Autodesk Inventor part; units mm, degrees
ref_plane "YZ Plane" through (0, 0, 0) normal (1, 0, 0) x (0, 1, 0)
ref_plane "XZ Plane" through (0, 0, 0) normal (0, 1, 0) x (-1, 0, 0)
ref_plane "XY Plane" through (0, 0, 0) normal (0, 0, 1) x (1, 0, 0)
sketch "Sketch1" plane through (0, 0, 0) normal (0, 0, 1) x (1, 0, 0)
  line L0 (-20, -12) -> (20, -12)
  line L1 (20, -12) -> (20, 12)
  line L2 (20, 12) -> (-20, 12)
  line L3 (-20, 12) -> (-20, -12)
  line L4 (-20, -12) -> (20, 12) construction
  line L5 (20, -12) -> (-20, 12) construction
  point P0 (0, 0)
  dimension "d0" = 40
  dimension "d1" = 24
extrude "Extrusion1" add sketch "Sketch1" along normal blind 45
sketch "Sketch2" plane through (0, 0, 45) normal (0, 0, 1) x (1, 0, 0)
  line L0 (-20, -6) -> (-19.2, -6)
  line L1 (-19.2, -6) -> (-19.2, 6)
  line L2 (-19.2, 6) -> (-20, 6)
  line L3 (-20, 6) -> (-20, -6)
  line L4 (20, -12) -> (20, 12)
  line L5 (20, -6) -> (19.2, -6)
  line L6 (19.2, -6) -> (19.2, 6)
  line L7 (19.2, 6) -> (20, 6)
  line L8 (20, 6) -> (20, -6)
  point P0 (0, 0)
  point P1 (-20, 12)
  point P2 (-19.2, 0)
  point P3 (19.2, 0)
  dimension "d4" = 12
  dimension "d5" = 0.8
  dimension "d6" = 0.8
extrude "Extrusion2" add sketch "Sketch2" along normal blind 2.5
sketch "Sketch3" plane through (20, -12, 0) normal (1, 0, 0) x (0, 0, -1)
  line L0 (-47.5, 6) -> (-47.5, 18)
  line L1 (-47.5, 18) -> (-46.7, 18)
  line L2 (-46.7, 18) -> (-46.7, 6)
  line L3 (-46.7, 6) -> (-47.5, 6)
  line L4 (-47.5, 6) -> (-47.5, 18)
  point P0 (0, 12)
  dimension "d9" = 0.8
extrude "Extrusion3" add sketch "Sketch3" along normal blind 14
sketch "Sketch4" plane through (-20, -12, 0) normal (-1, 0, 0) x (0, 0, 1)
  line L0 (47.5, 18) -> (47.5, 6)
  line L1 (45, 18) -> (47.5, 18)
  line L2 (47.5, 6) -> (46.7, 6)
  line L3 (46.7, 6) -> (46.7, 18)
  line L4 (46.7, 18) -> (47.5, 18)
  line L5 (47.5, 18) -> (47.5, 6)
  point P0 (0, 12)
  dimension "d12" = 0.8
extrude "Extrusion4" add sketch "Sketch4" along normal blind 14
sketch "Sketch5" plane through (0, 0, 47.5) normal (0, 0, 1) x (1, 0, 0)
  line L0 (-28, 0) -> (28, 0) construction
  point P0 (0, 0)
  point P1 (0, 0)
  dimension "d15" = 56
hole "Hole1" at (-28, 0, 47.5) at (28, 0, 47.5) direction (0, 0, -1) diameter 5.5 end through all
fillet "Fillet1" radius 1 2 edges at (19.2, 0, 47.5) (-19.2, 0, 47.5)
properties part number "Snmubber"
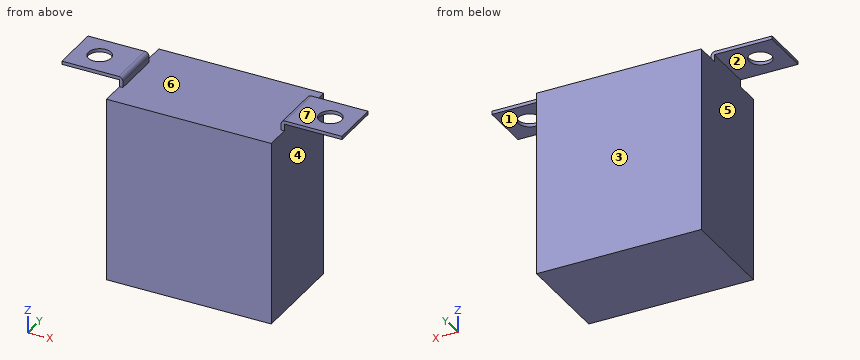
The listing builds one solid part. Answer for the finished solid, in the listing's coordinates (mm). Face numbers are marked on the shaded views. A direction names the side the tool comes from. Give positions to 0.01 mm unless a question says otherwise; leave off trailing zeros. Order: outer loops, then holes, each group sorted by start corner. A loop starts at its lowest first (then second) coordinate and runs counter-clockwise, first axis right, second up. Notation, with made-up numbers: (13, -10) - (40, -10) arc R12 cw to (40, 11) - close; hole circle Ø4 at (38, 54.25). An arc over 180 degrees is marked (long way). Answer in a Markdown table with one row per item. Add a question column.
Q1. The part is cut by section A-A (x = -28). Determine the outline of the cut face in (y, z), then the cut area to 3 significant figures.
Q2. The part is cut by section D-D (z = 41). Determine the outline of the cut face in (x, y).
Q3. Which of the six approach directions +Z, -Z, +X, -X, +Y, -Y give full straight-line access (tool end or side, diameter ignored) to the marked faces 1, 2 and 3?
Q4. For a pull along X with two mould halves and no side action, classify the marked faces 4, 5, 6 and 7 as released by +X, released by -X, zero draft, split by the parting line, or undercut.
Q5. The part is cut by section B-B (y = 0). Determine the outline of the cut face in (x, z), then the cut area to 3 significant figures.
Q6. Find the intervals of material crossed by line 1 along X through (y, z) = (0, 47.25); line 2 along Y through (x, z) = (28, 47.1); line 3 along X through (y, z) = (0, 47.1), in increasing order. Write a range as [from, to].
Q7. The part is cut by section C-C (y = -4.75). Determine the outline of the cut face in (x, z).
Q8. Given P1, Ø12, axis at y = -5.5, z = 23, coming from the +X side; P2, Ø0.8, axis at x = 23.5, z = 46, coming from the +Y side (1 decimal); P3, Ø7, axis at x = 28, y = 0, coming from the -Z side; P4, Ø12, axis at y = -1.5, z = 21, coming from the -X side, each flat-ended and moving along its own axis, determine where each tip first touches the part or whether it passes through.
Determined:
| question | item | result |
|---|---|---|
| 1 | outline | (-6, 46.7) - (-2.75, 46.7) - (-2.75, 47.5) - (-6, 47.5) - close; (2.75, 46.7) - (6, 46.7) - (6, 47.5) - (2.75, 47.5) - close |
| 1 | area | 5.20 mm² |
| 2 | outline | (-20, -12) - (20, -12) - (20, 12) - (-20, 12) - close |
| 3 | face 1 | -Z, +X, +Y, -Y |
| 3 | face 2 | -Z, -X, +Y, -Y |
| 3 | face 3 | +Z, -Z, +X, -X, +Y |
| 4 | face 4 | released by +X |
| 4 | face 5 | released by -X |
| 4 | face 6 | undercut |
| 4 | face 7 | zero draft |
| 5 | outline | (-34, 46.7) - (-30.75, 46.7) - (-30.75, 47.5) - (-34, 47.5) - close; (-25.25, 46.7) - (-20, 46.7) - (-20, 0) - (20, 0) - (20, 46.7) - (25.25, 46.7) - (25.25, 47.5) - (20.2, 47.5) arc R1 ccw to (19.2, 46.5) - (19.2, 45) - (-19.2, 45) - (-19.2, 46.5) arc R1 ccw to (-20.2, 47.5) - (-25.25, 47.5) - close; (30.75, 46.7) - (34, 46.7) - (34, 47.5) - (30.75, 47.5) - close |
| 5 | area | 1,820 mm² |
| 6 | line 1 | x = [-34, -30.75], [-25.25, -19.54], [19.54, 25.25], [30.75, 34] |
| 6 | line 2 | y = [-6, -2.75], [2.75, 6] |
| 6 | line 3 | x = [-34, -30.75], [-25.25, -19.4], [19.4, 25.25], [30.75, 34] |
| 7 | outline | (-34, 46.7) - (-20, 46.7) - (-20, 0) - (20, 0) - (20, 46.7) - (34, 46.7) - (34, 47.5) - (20.2, 47.5) arc R1 ccw to (19.2, 46.5) - (19.2, 45) - (-19.2, 45) - (-19.2, 46.5) arc R1 ccw to (-20.2, 47.5) - (-34, 47.5) - close |
| 8 | P1 | stops at x = 20 |
| 8 | P2 | passes through |
| 8 | P3 | stops at z = 46.7 |
| 8 | P4 | stops at x = -20 |
